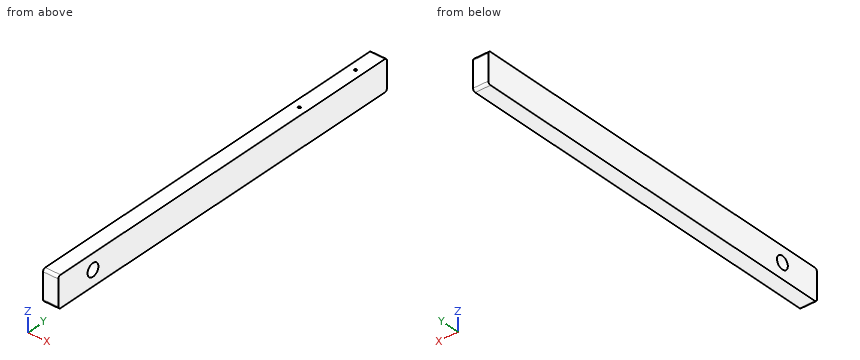
from build123d import *

# Parameters (mm, degrees)
F0_W     = 482.6
F0_H     = 38.1
F0_R     = 7.9375
F1_DEPTH = 9.525
F2_R     = 1.5875
F3_DEPTH = 25.4
F4_R     = 3.175
F5_R     = 3.175


with BuildPart() as f1:
    # F0 (on Right) → F1 (new body, symmetric)
    with BuildSketch(Plane.YZ):
        with Locations((190.5, 0)):
            Rectangle(F0_W, F0_H)
        Circle(F0_R, mode=Mode.SUBTRACT)
    extrude(amount=F1_DEPTH, both=True)

    # F2 (on face) → F3 (cut)
    with BuildSketch(Plane.XY.offset(19.05)):
        with Locations((0, 396.875)):
            Circle(F2_R)
        with Locations((0, 314.325)):
            Circle(F2_R)
    extrude(amount=-F3_DEPTH, mode=Mode.SUBTRACT)

    # F4
    f4_edges = [f1.edges().sort_by_distance(p)[0] for p in [
        (0, 431.8, -19.05),
    ]]
    fillet(f4_edges, radius=F4_R)

    # F5
    f5_edges = [f1.edges().sort_by_distance(p)[0] for p in [
        (0, 431.8, 19.05),
        (0, -50.8, -19.05),
        (0, -50.8, 19.05),
    ]]
    fillet(f5_edges, radius=F5_R)


solid = f1.part
Model file for the job. Use its own axes, mm. Coordinates: 2 decimals unless noted, no trailing zeros. Write each loop counter-clockwise with the first axis right and the second up, starting at its lowest first coordinate (ties: lowest second). Pieces come first, ordered by that corner, then holes. Notation, with made-up numbers: (74.5, 38.25) -> (102.5, 38.25) arc R21 ccw to (102.5, 62.25) -> close; hole circle Ø7 at (-20.5, 49.5). An arc over 180 degrees is marked (long way). One line per item, written item: value. Start each with the question number.
1) Flat gauge pins, fed straight in: pin 1 Ø1.6 at (x, y) = (0.5, 396.5) entering from +Z; pin 2 Ø3.5 at (x, y) = (-0.5, 314.5) entering from +Z. Where does each tip first touch, or does it go through?
2) Slice it at B-B on z = 0. Write the cut outline in (x, y) (1 decimal).
3) Probe probe 1 along Y at (x, z) = (0, 9); probe 2 along Y at (x, z) = (-6.5, -3); probe 3 along Y at (x, z) = (6, 4). List the from-to ranges inside material, lowest first.
Answers follow:
1. pin 1: z = -6.35
1. pin 2: z = 19.05
2. outline: (-9.5, -50.8) -> (9.5, -50.8) -> (9.5, -7.9) -> (-9.5, -7.9) -> close; (-9.5, 7.9) -> (9.5, 7.9) -> (9.5, 431.8) -> (-9.5, 431.8) -> close; hole circle Ø3.2 at (0, 314.3); hole circle Ø3.2 at (0, 396.9)
3. probe 1: -50.8 to 312.74, 315.91 to 395.29, 398.46 to 431.8
3. probe 2: -50.8 to -7.35, 7.35 to 431.8
3. probe 3: -50.8 to -6.86, 6.86 to 431.8
